Verification items for this drawing (mm, ordinates from the low corner). A direction names the side the tool comes from. Give positions to 0.01 mm unless a question says otherwise; leave off trailing zeros. Order: outer loops, then holes, each group sorted by start corner. A loop starts at its lowest first (then second) coordinate and runs counter-clockwise, first axis right, second up. Notation, with made-up numbers: M -39.5,70 L 12.5,70 A13 ccw 12.5,74 Z; hole C 4.5,-38.75 d11. An arc over 180 degrees is marked long. Answer as a JSON object with one key per item and string values.
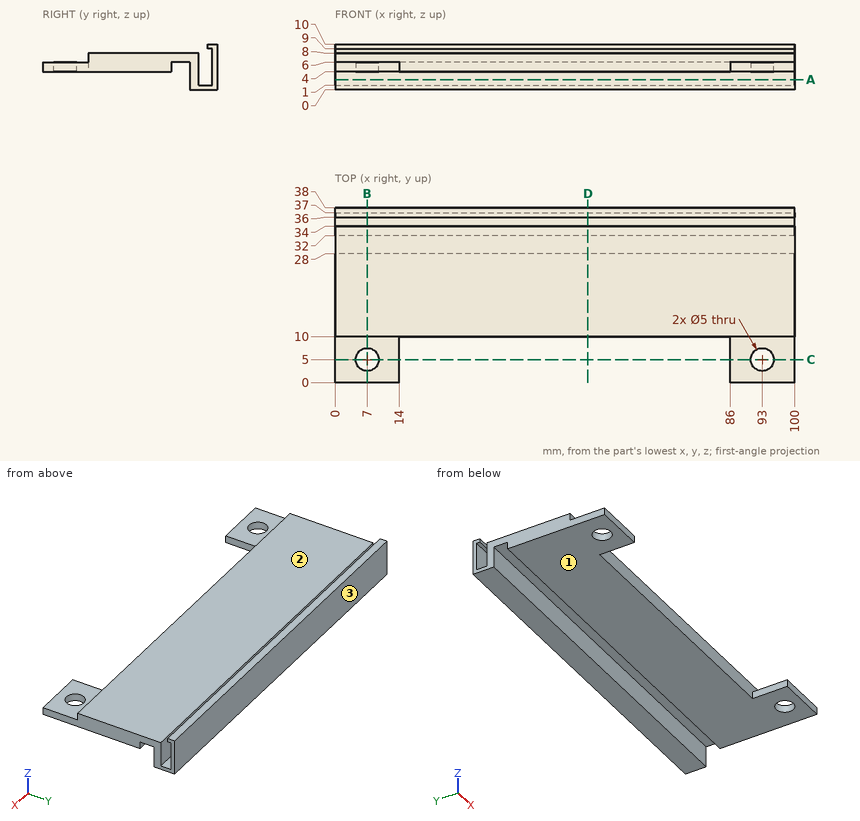
Q1. Material ranges on L1, parallel to Y at x = 93, z = 5.25; L2, parallel to Y at x = 73, z = 5; L3, parallel to X at y = 7, z = 4.75, recorded low to high.
Resolved:
{"L1": "y = 0 to 2.5, 7.5 to 28, 32 to 34, 37 to 38", "L2": "y = 10 to 28, 32 to 34, 37 to 38", "L3": "x = 0 to 5.5, 8.5 to 14, 86 to 91.5, 94.5 to 100"}
Q2. Section check C-C on y = 5. Record the cut outline in (x, z), then the cut area to 3 significant figures.
Resolved:
{"outline": "M 0,4 L 4.5,4 L 4.5,6 L 0,6 Z; M 9.5,4 L 14,4 L 14,6 L 9.5,6 Z; M 86,4 L 90.5,4 L 90.5,6 L 86,6 Z; M 95.5,4 L 100,4 L 100,6 L 95.5,6 Z", "area": "36.0 mm²"}
Q3. Section check A-A on z = 2.25. Record the cut outline in (x, y), then the cut area to 3 significant figures.
Resolved:
{"outline": "M 0,32 L 100,32 L 100,34 L 0,34 Z; M 0,37 L 100,37 L 100,38 L 0,38 Z", "area": "300 mm²"}
Q4. Gauge pin test, flat ends, axial feed: pin 1 Ø22.5 at (x, y) = (47.5, 9.5) entering from -Z; pin 2 Ø1.8 at (x, z) = (71, 3) entering from -Y; pin 3 Ø6 at (x, z) = (19, 5.5) entering from -Y; pin 4 Ø4 at (y, z) = (24.5, 4) entering from -X. Record the tip position at first contact, or that the pin passes through.
Resolved:
{"pin 1": "stops at z = 4", "pin 2": "stops at y = 32", "pin 3": "stops at y = 10", "pin 4": "stops at x = 0"}
Q5. Section check D-D on x = 55. Record the cut outline in (y, z).
Resolved:
{"outline": "M 10,4 L 28,4 L 28,6 L 32,6 L 32,0 L 38,0 L 38,10 L 36,10 L 36,9 L 37,9 L 37,1 L 34,1 L 34,8 L 10,8 Z"}
Q6. Section check B-B on x = 7. Record the cut outline in (y, z), then the cut area to 3 significant figures.
Resolved:
{"outline": "M 0,4 L 2.5,4 L 2.5,6 L 0,6 Z; M 7.5,4 L 28,4 L 28,6 L 32,6 L 32,0 L 38,0 L 38,10 L 36,10 L 36,9 L 37,9 L 37,1 L 34,1 L 34,8 L 10,8 L 10,6 L 7.5,6 Z", "area": "120 mm²"}
Q7. Tool access check on the marked faces 1, 2 and 3. Record the directions out of +Z, -Z, +X, -X, +Y, -Y that give a thin tool (end or side, any length) a straight path to the whole face; none if there is none.
Resolved:
{"face 1": "-Z, +X, -X, -Y", "face 2": "+Z, +X, -X, -Y", "face 3": "+Z, -Z, +X, -X, +Y"}
